```python
from build123d import *

# Parameters (mm, degrees)
EXTRUDE_1_DEPTH       = 245
EXTRUDE_3_DEPTH       = 245
PATTERN_CURVE_1_COUNT = 19
PATTERN_CURVE_1_PITCH = 9.75
SKETCH_7_R            = 2.6
CUT_EXTRUDE_4_DEPTH   = 6
CUT_EXTRUDE_START     = -8
SKETCH_13_R           = 2.6
CUT_EXTRUDE_9_DEPTH   = 8
SKETCH_15_R           = 1.6
SKETCH_15_R_2         = 1.3
SKETCH_15_R_3         = 2.6
CUT_EXTRUDE_10_DEPTH  = 10


with BuildPart() as part:
    # Эскиз1 → Вытянуть1 (new body)
    with BuildSketch(Plane.XY):
        with BuildLine():
            Line((0, 45), (2.564446908, 45))
            ThreePointArc((2.564446908, 45), (3.247630994, 44.730246195), (3.562232066, 44.066519011))
            Line((3.562232066, 44.066519011), (5.5, 15))
            Line((5.5, 15), (194.5, 15))
            Line((194.5, 15), (196.437767934, 44.066519011))
            ThreePointArc((196.437767934, 44.066519011), (196.752369006, 44.730246195), (197.435553092, 45))
            Line((197.435553092, 45), (200, 45))
            Line((200, 45), (200, 0))
            Line((200, 0), (0, 0))
            Line((0, 0), (0, 45))
        make_face()
    extrude(amount=EXTRUDE_1_DEPTH)

    # Эскиз2 → Вытянуть3 (add)
    with BuildSketch(Plane.XY.offset(245)):
        with BuildLine():
            Line((11.5, 44.5), (10, 15))
            Line((10, 15), (14, 15))
            Line((14, 15), (12.5, 44.5))
            ThreePointArc((12.5, 44.5), (12, 45), (11.5, 44.5))
        make_face()
    extrude_3 = extrude(amount=-EXTRUDE_3_DEPTH)

    # Кривая1: Вытянуть3 ×19
    with Locations(*[(i * PATTERN_CURVE_1_PITCH, 0, 0) for i in range(1, PATTERN_CURVE_1_COUNT)]):
        add(extrude_3)

    # Эскиз7 → Вырез-Вытянуть4 (cut)
    with BuildSketch(Plane.ZY):
        with Locations(Location((22.5, 20, 0), (0, 0, 270))):
            Circle(SKETCH_7_R)
        with Locations(Location((222.5, 20, 0), (0, 0, 270))):
            Circle(SKETCH_7_R)
        with Locations(Location((122.5, 20, 0), (0, 0, 270))):
            Circle(SKETCH_7_R)
    extrude(amount=-CUT_EXTRUDE_4_DEPTH, mode=Mode.SUBTRACT)

    # Эскиз13 → Вырез-Вытянуть9 (cut)
    with BuildSketch(Plane(origin=(200, 0, 0), x_dir=(0, 0, -1), z_dir=(1, 0, 0)).offset(CUT_EXTRUDE_START)):
        with Locations(Location((-222.5, 20, 0), (0, 0, 270))):
            Circle(SKETCH_13_R)
        with Locations(Location((-122.5, 20, 0), (0, 0, 270))):
            Circle(SKETCH_13_R)
        with Locations(Location((-22.5, 20, 0), (0, 0, 270))):
            Circle(SKETCH_13_R)
    extrude(amount=CUT_EXTRUDE_9_DEPTH, mode=Mode.SUBTRACT)

    # Эскиз15 → Вырез-Вытянуть10 (cut)
    with BuildSketch(Plane.XZ):
        with Locations((25, 220)):
            Circle(SKETCH_15_R)
        with Locations((175, 220)):
            Circle(SKETCH_15_R)
        with Locations((175, 110)):
            Circle(SKETCH_15_R)
        with Locations((25, 110)):
            Circle(SKETCH_15_R)
        with Locations((55, 182)):
            Circle(SKETCH_15_R_2)
        with Locations((55, 148.5)):
            Circle(SKETCH_15_R_2)
        with Locations((93, 195)):
            Circle(SKETCH_15_R_3)
    extrude(amount=-CUT_EXTRUDE_10_DEPTH, mode=Mode.SUBTRACT)


solid = part.part
```
Part model, mm, in its own coordinate system. A direction names the side the tool comes from. Round coordinates to 2 decimals unless told otherwise and drop trailing zeros. Use CSV: the item, a comma, the result in double quotes. Start each with the question number.
1) Pull direction Z, two halves, no side cores. Call faces 1 (the flat face through (101, 18, 0)), 2 (the cylindrical face through (2.63, 17.52, 123.28)), 3 (the flat face through (42.51, 29.54, 124.22)): +Z half, -Z half, draft (parallel to the pull), parting line (faces both ways), or undercut.
2) Drop flat-ended pins along their axis: P1, Ø1.7, axis at x = 183.5, z = 103.5, coming from the +Y side; P2, Ø6.5, axis at x = 103, z = 133, coming from the +Y side; P3, Ø2, axis at x = 74.5, y = 22.5, coming from the +Z side; P4, Ø1.6, axis at x = 93.5, z = 195, coming from the -Y side. Give the stop position or say it passes through.
3) Cut at A-A, the plane y = 31.5. Give the number of separate pieces and of enclosed holes in the cut face, plus the area to 3 significant figures.
4) Which spindle directions (+Z, -Z, +X, -X, +Y, -Y) get a long thin tool onto all of the face, cutting with end or side? Do faces 4 (the cylindrical face through (2.63, 17.52, 23.28)), 5 (the flat face through (101, 0, 121)), 6 (the flat face through (79.01, 29.96, 124.22)). Say none if no direction does.
5) Wall check: L1, parallel to Z at x = 25, y = 2; L2, parallel to Z at x = 93, y = 5; L3, parallel to Y at x = 197.6, z = 22.5. Give the ranges that are in metal, low to high. Write a range as [from, to].
Determined:
1,face 1,"-Z half"
1,face 2,"undercut"
1,face 3,"draft"
2,P1,"stops at y = 15"
2,P2,"stops at y = 45"
2,P3,"passes through"
2,P4,"stops at y = 10"
3,separate pieces,"21"
3,enclosed holes,"0"
3,area,"13,000 mm2"
4,face 4,"-X"
4,face 5,"+Z, -Z, +X, -X, -Y"
4,face 6,"+Z, -Z, +Y"
5,L1,"z = [0, 108.4], [111.6, 218.4], [221.6, 245]"
5,L2,"z = [0, 192.4], [197.6, 245]"
5,L3,"y = [0, 17.4], [22.6, 45]"
